```python
from build123d import *

# Parameters (mm, degrees)
SKETCH1_R                = 22.5
SKETCH1_R_2              = 15
SKETCH1_R_3              = 2
BOSS_EXTRUDE1_DEPTH      = 5
BOSS_EXTRUDE2_DEPTH      = 10
BOSS_EXTRUDE2_DEPTH_BACK = 2.5
SKETCH1_2_R              = 15
SKETCH4_R                = 2
SKETCH4_R_2              = 15
BOSS_EXTRUDE3_DEPTH      = 5
SKETCH4_3_R              = 15
SKETCH4_3_R_2            = 10
BOSS_EXTRUDE4_DEPTH      = 12.5
SWEEP3_PROFILE_R         = 15
BOSS_EXTRUDE5_DEPTH      = 4.99
SKETCH24_R               = 10


with BuildPart() as part:
    # Sketch1 → Boss-Extrude1 (new body)
    with BuildSketch(Plane.XY):
        Circle(SKETCH1_R)
        Circle(SKETCH1_R_2, mode=Mode.SUBTRACT)
        with Locations((13.081475452, 13.081475452)):
            Circle(SKETCH1_R_3, mode=Mode.SUBTRACT)
        with Locations(Location((-13.081475452, 13.081475452, 0), (0, 0, 180))):
            Circle(SKETCH1_R_3, mode=Mode.SUBTRACT)
        with Locations((-13.081475452, -13.081475452)):
            Circle(SKETCH1_R_3, mode=Mode.SUBTRACT)
        with Locations(Location((13.081475452, -13.081475452, 0), (0, 0, 180))):
            Circle(SKETCH1_R_3, mode=Mode.SUBTRACT)
    extrude(amount=BOSS_EXTRUDE1_DEPTH)

    # Sketch1_2 → Boss-Extrude2 (add, two sides: drawn at the far end of the back side and taken through both)
    with BuildSketch(Plane.XY.offset(-BOSS_EXTRUDE2_DEPTH_BACK)):
        Circle(SKETCH1_2_R)
    extrude(amount=BOSS_EXTRUDE2_DEPTH + BOSS_EXTRUDE2_DEPTH_BACK)



with BuildPart() as body_2:
    # Sketch4 → Boss-Extrude3 (new body)
    with BuildSketch(Plane(origin=(-59.111206886, 0, 21.514719818), x_dir=(0, -1, 0), z_dir=(-0.9396926207859094, 0, 0.34202014332566616))):
        with BuildLine():
            ThreePointArc((-20, 53.746291113), (-18.828427125, 56.574718238), (-16, 57.746291113))
            Line((-16, 57.746291113), (16, 57.746291113))
            ThreePointArc((16, 57.746291113), (18.828427125, 56.574718238), (20, 53.746291113))
            Line((20, 53.746291113), (20, 21.746291113))
            ThreePointArc((20, 21.746291113), (18.828427125, 18.917863989), (16, 17.746291113))
            Line((16, 17.746291113), (-16, 17.746291113))
            ThreePointArc((-16, 17.746291113), (-18.828427125, 18.917863989), (-20, 21.746291113))
            Line((-20, 21.746291113), (-20, 53.746291113))
        make_face()
        with Locations(Location((-16, 21.746291113, 0), (0, 0, 90))):
            Circle(SKETCH4_R, mode=Mode.SUBTRACT)
        with Locations(Location((-16, 53.746291113, 0), (0, 0, 90))):
            Circle(SKETCH4_R, mode=Mode.SUBTRACT)
        with Locations(Location((16, 53.746291113, 0), (0, 0, 90))):
            Circle(SKETCH4_R, mode=Mode.SUBTRACT)
        with Locations(Location((0, 37.746291113, 0), (0, 0, 90))):
            Circle(SKETCH4_R_2, mode=Mode.SUBTRACT)
        with Locations(Location((16, 21.746291113, 0), (0, 0, 90))):
            Circle(SKETCH4_R, mode=Mode.SUBTRACT)
    extrude(amount=-BOSS_EXTRUDE3_DEPTH)

    # Sketch4_3 → Boss-Extrude4 (add)
    # profile 1 of 2: a face of its own
    with BuildSketch(Plane(origin=(-59.111206886, 0, 21.514719818), x_dir=(0, -1, 0), z_dir=(-0.9396926207859094, 0, 0.34202014332566616))):
        with Locations(Location((0, 37.746291113, 0), (0, 0, 90))):
            Circle(SKETCH4_3_R)
        with Locations((0, 37.746291113)):
            Circle(SKETCH4_3_R_2, mode=Mode.SUBTRACT)
    # profile 2 of 2: a face of its own
    with BuildSketch(Plane(origin=(-59.111206886, 0, 21.514719818), x_dir=(0, -1, 0), z_dir=(-0.9396926207859094, 0, 0.34202014332566616))):
        with Locations((0, 37.746291113)):
            Circle(SKETCH4_3_R_2)
    extrude(amount=-BOSS_EXTRUDE4_DEPTH)


with BuildPart() as part_1:
    add(part.part)

    add(body_2.part)  # Sweep3 merges body 2
    # Sweep3: sweep along a curve in space
    with BuildLine() as sweep3_path:
        ThreePointArc((0, 0, 10), (-10.844948453, 0, 36.503726407), (-34.45505723, 0, 52.709379248))
    # Sweep3 profile (on start of the path) → Sweep3 (sweep)
    with BuildSketch(Plane(origin=(0, 0, 10), x_dir=(0.9952050551288538, 0, 0.09781052216390201), z_dir=(-0.09781052216390201, 0, 0.9952050551288538))):
        Circle(SWEEP3_PROFILE_R)
    sweep(path=sweep3_path.line)

    # Sketch22 → Boss-Extrude5 (add)
    with BuildSketch(Plane.XZ.offset(20)):
        with BuildLine():
            Line((-32.231926298, 58.817381283), (-39.279620954, 61.382532358))
            Line((-39.279620954, 61.382532358), (-43.725882817, 49.166528288))
            Line((-43.725882817, 49.166528288), (-36.678188161, 46.601377213))
            ThreePointArc((-36.678188161, 46.601377213), (-40.563059265, 54.932510179), (-32.231926298, 58.817381283))
        make_face()
        with BuildLine():
            ThreePointArc((-27.95505723, 52.709379248), (-29.130568942, 56.437626084), (-32.231926298, 58.817381283))
            Line((-32.231926298, 58.817381283), (-33.4289968, 55.52845711))
            ThreePointArc((-33.4289968, 55.52845711), (-31.997601097, 54.430108557), (-31.45505723, 52.709379248))
            ThreePointArc((-31.45505723, 52.709379248), (-32.734327921, 50.251923115), (-35.48111766, 49.890301385))
            Line((-35.48111766, 49.890301385), (-36.678188161, 46.601377213))
            ThreePointArc((-36.678188161, 46.601377213), (-30.726810394, 47.38489096), (-27.95505723, 52.709379248))
        make_face()
        with BuildLine():
            Line((-33.4289968, 55.52845711), (-32.231926298, 58.817381283))
            ThreePointArc((-32.231926298, 58.817381283), (-40.563059265, 54.932510179), (-36.678188161, 46.601377213))
            Line((-36.678188161, 46.601377213), (-35.48111766, 49.890301385))
            ThreePointArc((-35.48111766, 49.890301385), (-37.274135092, 53.735439678), (-33.4289968, 55.52845711))
        make_face()
    extrude(amount=-BOSS_EXTRUDE5_DEPTH)

    # Sketch24 → Cut-Revolve1 (revolve, cut)
    with BuildSketch(Plane.XY.offset(10), mode=Mode.PRIVATE) as cut_revolve1_sk:
        Circle(SKETCH24_R)
    revolve(cut_revolve1_sk.sketch.rotate(Axis((-50, 66.423618384, 10), (0, -1, 0)), 26.245287908), axis=Axis((-50, 66.423618384, 10), (0, -1, 0)), mode=Mode.SUBTRACT)


solid = part_1.part
```
CAD build for the part. Positions are in the model's coordinates, mm. A direction names the side the tool comes from. Coordinates: 2 decimals unless noted, no trailing zeros. Use CSV: the item, a comma, the result in double quotes. Start each with the question number.
Q1. Drop flat-ended pins along their axis: P1, Ø1.5, axis at x = -24.5, y = 12, coming from the +Z side; P2, Ø7.5, axis at x = 5, y = 4.5, coming from the +Z side; P3, Ø19, axis at x = -38.5, z = 53.5, coming from the -Y side. Give the stop position or say it passes through.
Q2. Two-plate mould, pull along Y, no slides. Class faces 5 (the cylindrical face through (-14.985, 0.66, -1.268)), 6 (the cylindrical face through (-14.99, 12.48, 2.46)), 7 (the flat face through (-40.25, -17.54, 47.9)): +Y half, -Y half, draft (parallel to the pull), parting line (faces both ways), or undercut.
Q3. Cut at A-A, the plane y = 0. State how many separate pieces and enclosed holes the cut face has, then the cut area to 3 significant figures.
Q4. 3-axis set-ups, long thin cutter, end or side, ignore diameter. For faces 1 (the flat face through (-49.146, -0.28, 48.895)), 2 (the cylindrical face through (-12, -11.4, 2.5)), 3 (the cylindrical face through (13.856, -5.745, 7.465)), 4 (the flat face through (-35.706, -17.54, 60.082)): which of +Z, -Z, +X, -X, +Y, -Y reach the whole face in a straight line?
Q5. Probe probe 1 along Y at (x, z) = (0, 13.5); probe 2 along Z at (x, y) = (7.5, -15); probe 3 along Y at (x, z) = (-15.5, 57). List the from-to ranges inside material, lowest first. Write a range as from..to.
Here are the results:
1,P1,"z = 59.51"
1,P2,"z = 44.55"
1,P3,"y = -20"
2,face 5,"parting line"
2,face 6,"undercut"
2,face 7,"draft"
3,separate pieces,"4"
3,enclosed holes,"0"
3,area,"880 mm2"
4,face 1,"+Z, -X, +Y, -Y"
4,face 2,"-Z"
4,face 3,"none"
4,face 4,"+X, -Y"
5,probe 1,"-14.99..-10, 10..14.99"
5,probe 2,"0..5"
5,probe 3,"-8.75..-5.57, 5.57..8.75"
